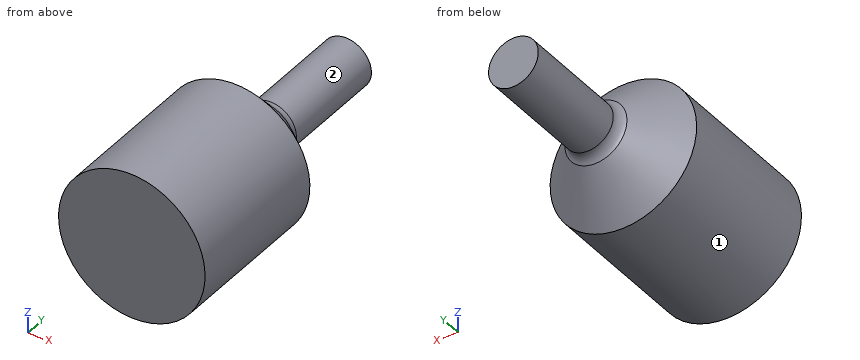
from build123d import *

# Parameters (mm, degrees)
SKETCH1_R           = 2.95
BOSS_EXTRUDE1_DEPTH = 7.7
SKETCH3_R           = 1
BOSS_EXTRUDE2_DEPTH = 4.8
FILLET1_R           = 0.5


with BuildPart() as part:
    # Sketch1 → Boss-Extrude1 (new body)
    with BuildSketch(Plane(origin=(0, 0, 0), x_dir=(1, 0, 0), z_dir=(0, 1, 0))):
        with Locations(Location((0, 0, 0), (0, 0, 90))):
            Circle(SKETCH1_R)
    extrude(amount=BOSS_EXTRUDE1_DEPTH)

    # Sketch2 → Cut-Revolve1 (revolve, cut)
    with BuildSketch(Plane.XY, mode=Mode.PRIVATE) as cut_revolve1_sk:
        Polygon((-2.95, 6.1), (-1.25, 7.7), (-2.95, 7.7), align=None)
    revolve(cut_revolve1_sk.sketch.rotate(Axis((0, 7.7, 0), (0, -1, 0)), 90), axis=Axis((0, 7.7, 0), (0, -1, 0)), mode=Mode.SUBTRACT)

    # Sketch3 → Boss-Extrude2 (add)
    with BuildSketch(Plane(origin=(0, 7.7, 0), x_dir=(1, 0, 0), z_dir=(0, 1, 0))):
        with Locations(Location((0, 0, 0), (0, 0, 270))):
            Circle(SKETCH3_R)
    extrude(amount=BOSS_EXTRUDE2_DEPTH)

    # Fillet1
    # the kernel refuses this fillet: 0.5 mm, written as the material it adds along each edge
    with BuildSketch(Plane(origin=(0, 7.7, 0), x_dir=(0, 0, 1), z_dir=(-1, 0, 0))) as fillet1_piece_1:
        with BuildLine():
            CenterArc((1.5, 0.433012702), FILLET1_R, 180, 60)
            Line((1, 0.433012702), (0.99, 0.433012702))
            Line((0.99, 0.433012702), (0.99, 0))
            Line((0.99, 0), (1, -0.01))
            ThreePointArc((1, -0.01), (1.125, -0.01), (1.245, -0.008660254))
            Line((1.245, -0.008660254), (1.25, 0))
        make_face()
    revolve(axis=Axis((0, 7.7, 0), (0, 1, 0)))


solid = part.part
Geometry check sheet. Reference: the model listing, model coordinates, mm. Face numbers are marked on the shaded views. A direction names the side the tool comes from. Coordinates: 2 decimals unless noted, no trailing zeros. Order: outer loops, then holes, each group sorted by start corner. A loop starts at its lowest first (then second) coordinate and runs counter-clockwise, first axis right, second up. Notation, with made-up numbers: (76, 53.5) -> (87, 53.5) arc R26 ccw to (87, 67.5) -> close; hole circle Ø7 at (-31.75, 86.25). An arc over 180 degrees is marked (long way). Use a Markdown table: item, result. Add a question column.
1. Cross-section at D-D (y = 6.25). Enter the section's corners in (x, z), and give its area (3 significant figures).
2. Set-up check for the marked faces 1 and 2: record each of +Z, -Z, +X, -X, +Y, -Y from which the full face is reachable in a straight line by a thin tool's end or side.
3. Cross-section at B-B (z = 0). Enter the section's corners in (x, y).
4. Material ranges on L1, parallel to Z at x = -0.1, y = 2; L2, parallel to X at y = 8.25, z = 0.05; L3, parallel to Y at x = 0.25, z = 2.35, recorded low to high.
5. Cross-section at C-C (y = 2.75). Enter the section's corners in (x, z).
6. Go/stop test with flat-tipped pins: pin 1 Ø1 at (y, z) = (6.5, 2) entering from +X; pin 2 Ø2 at (x, y) = (-1.5, 10) entering from +Z; pin 3 Ø1.5 at (x, y) = (0.5, 9.5) entering from +Z. Record where each tip stops, or that it passes through.
7. Cross-section at A-A (x = 0). Enter the section's corners in (y, z), and give its area (3 significant figures).
Filled sheet:
| question | item | result |
|---|---|---|
| 1 | outline | circle Ø5.58 at (0, 0) |
| 1 | area | 24.5 mm2 |
| 2 | face 1 | +Y, -Y |
| 2 | face 2 | +Y |
| 3 | outline | (-2.95, 0) -> (2.95, 0) -> (2.95, 6.1) -> (1.25, 7.7) arc R0.5 cw to (1, 8.13) -> (1, 12.5) -> (-1, 12.5) -> (-1, 8.13) arc R0.5 cw to (-1.25, 7.7) -> (-2.95, 6.1) -> close |
| 4 | L1 | -2.95 to 2.95 |
| 4 | L2 | -1 to 1 |
| 4 | L3 | 0 to 6.65 |
| 5 | outline | circle Ø5.9 at (0, 0) |
| 6 | pin 1 | x = 2.41 |
| 6 | pin 2 | z = 0.87 |
| 6 | pin 3 | z = 1 |
| 7 | outline | (0, -2.95) -> (6.1, -2.95) -> (7.7, -1.25) arc R0.5 cw to (8.13, -1) -> (12.5, -1) -> (12.5, 1) -> (8.13, 1) arc R0.5 cw to (7.7, 1.25) -> (6.1, 2.95) -> (0, 2.95) -> close |
| 7 | area | 52.4 mm2 |
